CAD build for the part. Positions are in the model's coordinates, mm. A direction names the side the tool comes from. Round coordinates to 2 decimals unless told otherwise and drop trailing zeros. Order: outer loops, then holes, each group sorted by start corner. A loop starts at its lowest first (then second) coordinate and runs counter-clockwise, first axis right, second up. Notation, with made-up numbers: (4, -15) - (16, -15) arc R9 cw to (16, 2) - close; hole circle Ø3 at (22, 47.25). An arc over 180 degrees is marked (long way). Write item = value, one per line.
from build123d import *

# Parameters (mm, degrees)
BOSS_EXTRUDE1_DEPTH     = 35
CUT_EXTRUDE1_DEPTH      = 15.5
CUT_EXTRUDE1_DEPTH_BACK = 9.5
CUT_EXTRUDE2_DEPTH      = 51.214539727
CUT_EXTRUDE2_DEPTH_BACK = 51.214539727
SKETCH5_R               = 3
SKETCH5_W               = 35
SKETCH5_H               = 20
FILLET1_R               = 2
CUT_EXTRUDE3_DEPTH      = 51.214539727
CUT_EXTRUDE3_DEPTH_BACK = 51.214539727
SKETCH6_R               = 4


with BuildPart() as part:
    # Sketch1 → Boss-Extrude1 (new body)
    with BuildSketch(Plane(origin=(0, 0, 0), x_dir=(1, 0, 0), z_dir=(0, 1, 0))):
        Polygon((-32.5, 12.5), (32.5, 12.5), (32.5, 9.5), (5, -15.5), (-5, -15.5), (-32.5, 9.5), align=None)
    extrude(amount=BOSS_EXTRUDE1_DEPTH)

    # Sketch4 → Cut-Extrude1 (cut, two sides: drawn at the far end of the back side and taken through both)
    with BuildSketch(Plane.XY.offset(-CUT_EXTRUDE1_DEPTH_BACK)):
        Polygon((-23.214285714, 30), (23.214285714, 5), (32.5, 5), (32.5, 30), align=None)
        Polygon((-32.5, 5), (23.214285714, 5), (-23.214285714, 30), (-32.5, 30), align=None)
    extrude(amount=CUT_EXTRUDE1_DEPTH + CUT_EXTRUDE1_DEPTH_BACK, mode=Mode.SUBTRACT)

    # Sketch5 → Cut-Extrude2 (cut, two sides: drawn at the far end of the back side and taken through both)
    with BuildSketch(Plane.XY.offset(-CUT_EXTRUDE2_DEPTH_BACK)):
        with Locations((-25, 17.5)):
            Circle(SKETCH5_R)
        with Locations((25, 17.5)):
            Circle(SKETCH5_R)
        with Locations((0, 17.5)):
            Rectangle(SKETCH5_W, SKETCH5_H)
    extrude(amount=CUT_EXTRUDE2_DEPTH + CUT_EXTRUDE2_DEPTH_BACK, mode=Mode.SUBTRACT)

    # Fillet1
    fillet1_edges = [part.edges().sort_by_distance(p)[0] for p in [
        (17.5, 27.5, -11),
        (17.5, 7.5, -11),
        (-17.5, 7.5, -11),
        (-17.5, 27.5, -11),
    ]]
    fillet(fillet1_edges, radius=FILLET1_R)

    # Sketch6 → Cut-Extrude3 (cut, two sides: drawn at the far end of the back side and taken through both)
    with BuildSketch(Plane(origin=(0, 35, 0), x_dir=(1, 0, 0), z_dir=(0, 1, 0)).offset(-CUT_EXTRUDE3_DEPTH_BACK)):
        with Locations(Location((0, 1.5, 0), (0, 0, 270))):
            Circle(SKETCH6_R)
    extrude(amount=CUT_EXTRUDE3_DEPTH + CUT_EXTRUDE3_DEPTH_BACK, mode=Mode.SUBTRACT)


solid = part.part
(1) Drop a flat-ended pin along its axis: pin 1 (7 mm diameter, centred on x = 0, z = -1.5, fed in from -Y). Give the stop position or say it passes through.
Solved:
pin_1 = through
(2) Band-saw the part on B-B on z = -1.5. List the corners of the cut face in (x, y), plus the area to 3 significant figures.
Solved:
outline = (-23.7, 0) - (-4, 0) - (-4, 5) - (-23.7, 5) - close; (-23.7, 30) - (-4, 30) - (-4, 35) - (-23.7, 35) - close; (4, 0) - (23.7, 0) - (23.7, 5) - (4, 5) - close; (4, 30) - (23.7, 30) - (23.7, 35) - (4, 35) - close
area = 394 mm²
(3) Band-saw the part on A-A on y = 24.5. List the corners of the cut face in (x, z).
Solved:
outline = (-32.5, -12.5) - (-17.5, -12.5) - (-17.5, -9.5) - (-32.5, -9.5) - close; (17.5, -12.5) - (32.5, -12.5) - (32.5, -9.5) - (17.5, -9.5) - close
(4) Band-saw the part on C-C on x = 0. List the corners of the cut face in (y, z), plus the area to 3 significant figures.
Solved:
outline = (0, -12.5) - (7.5, -12.5) - (7.5, -9.5) - (5, -9.5) - (5, -5.5) - (0, -5.5) - close; (0, 2.5) - (5, 2.5) - (5, 15.5) - (0, 15.5) - close; (27.5, -12.5) - (35, -12.5) - (35, -5.5) - (30, -5.5) - (30, -9.5) - (27.5, -9.5) - close; (30, 2.5) - (35, 2.5) - (35, 15.5) - (30, 15.5) - close
area = 215 mm²
(5) Probe line 1 along X through (y, z) = (17.5, -10.9); line 2 along Z through (x, y) = (0, 2); line 3 along Y through (x, z) = (-21, -3.75). List the from-to ranges inside material, lowest first.
Solved:
line_1 = -32.5 to -28, -22 to -17.5, 17.5 to 22, 28 to 32.5
line_2 = -12.5 to -5.5, 2.5 to 15.5
line_3 = 0 to 5, 30 to 35
(6) Band-saw the part on D-D on y = 17.5. List the corners of the cut face in (x, z), plus the area to 3 significant figures.
Solved:
outline = (-32.5, -12.5) - (-28, -12.5) - (-28, -9.5) - (-32.5, -9.5) - close; (-22, -12.5) - (-17.5, -12.5) - (-17.5, -9.5) - (-22, -9.5) - close; (17.5, -12.5) - (22, -12.5) - (22, -9.5) - (17.5, -9.5) - close; (28, -12.5) - (32.5, -12.5) - (32.5, -9.5) - (28, -9.5) - close
area = 54.0 mm²
(7) Tool access for faces 1 (the cylindrical face through (-16.93, 26.9, -10.98)), 2 (the flat face through (0, 5, 3)), 3 (the flat face through (-18.558, 32.465, 3.175)): list every direction of +Z, -Z, +X, -X, +Y, -Y with a clear straight run to the whole face (end or side of a thin tool).
Solved:
face_1 = +Z, -Z
face_2 = +Z, +X, -X
face_3 = +Z, -X, +Y, -Y
(8) Pull direction Y, two halves, no side cores. Call faces 4 (the flat face through (0, 2, 15.5)), 5 (the cylindrical face through (-25.65, 14.57, -11.02)), 6 (the flat face through (0, 35, -8)): released by +Y, released by -Y, zero draft, split by the parting line, or undercut.
Solved:
face_4 = zero draft
face_5 = undercut
face_6 = released by +Y
